```python
from build123d import *

# Parameters (mm, degrees)
F1_DEPTH       = 3.81
F2_R           = 0.254
F3_D           = 1.778
F3_CSINK_D     = 3.175
F3_CSINK_ANGLE = 82


# Not quite as in the source:
# - a feature names something its author has since deleted; it is built from what else it names


with BuildPart() as f1:
    # F0 (on Front) → F1 (new body)
    with BuildSketch(Plane.XZ):
        with BuildLine():
            ThreePointArc((-15.3976073489, 30.0757028162), (-12.6205023663, 18.8138288447), (-15.6854130328, 7.6268524863))
            ThreePointArc((-15.6854130328, 7.6268524863), (-31.3905262472, 3.5144175537), (-39.2854884267, 17.7000537515))
            ThreePointArc((-39.2854884267, 17.7000537515), (-40.2547680717, 20.6965618199), (-43.3147661388, 21.4415285736))
            ThreePointArc((-43.3147661388, 21.4415285736), (-45.5440273695, 15.8957464039), (-45.905020088, 9.9295927212))
            ThreePointArc((-45.905020088, 9.9295927212), (-45.0345404234, 3.597348812), (-45.905020088, -2.7348950971))
            ThreePointArc((-45.905020088, -2.7348950971), (-45.1259294206, -6.5201466433), (-41.5899753571, -8.0796787515))
            Line((-41.5899753571, -8.0796787515), (-40.2320445972, -8.0796787515))
            Line((-40.2320445972, -8.0796787515), (-40.5776619182, -3.1953468446))
            Line((-40.5776619182, -3.1953468446), (-40.0765932374, -1.5246287875))
            Line((-40.0765932374, -1.5246287875), (-40.6392291188, -1.5644411324))
            Line((-40.6392291188, -1.5644411324), (-40.6392291188, 0.5960793933))
            Line((-40.6392291188, 0.5960793933), (-40.0844532998, 0.5960793933))
            Line((-40.0844532998, 0.5960793933), (-40.0844532998, 1.8968694892))
            ThreePointArc((-40.0844532998, 1.8968694892), (-36.1157211919, 2.6708049351), (-32.1480344873, 1.8915278128))
            ThreePointArc((-32.1480344873, 1.8915278128), (-26.4720596319, 0.9912977201), (-20.7960847765, 1.8915278128))
            ThreePointArc((-20.7960847765, 1.8915278128), (-16.7308465178, 3.8739299722), (-13.7448431924, 7.2709675878))
            ThreePointArc((-13.7448431924, 7.2709675878), (-12.3233048625, 12.470180408), (-11.6768007285, 17.821312772))
            ThreePointArc((-11.6768007285, 17.821312772), (-12.1024444853, 23.5936908911), (-13.2695324719, 29.2628555023))
            ThreePointArc((-13.2695324719, 29.2628555023), (-12.6323011565, 32.3319998397), (-9.8052835092, 33.6861349642))
            ThreePointArc((-9.8052835092, 33.6861349642), (-11.5106118889, 35.4421925399), (-12.2696207836, 37.7693772316))
            ThreePointArc((-12.2696207836, 37.7693772316), (-13.3462306374, 38.3418830024), (-13.8277616352, 39.4621416926))
            ThreePointArc((-13.8277616352, 39.4621416926), (-14.9168802382, 39.2283992754), (-15.6854130328, 38.4220667183))
            ThreePointArc((-15.6854130328, 38.4220667183), (-16.3374101507, 34.221439938), (-15.3976073489, 30.0757028162))
        make_face()
    extrude(amount=F1_DEPTH)

    # F2
    f2_edges = [f1.edges().sort_by_distance(p)[0] for p in [
        (-45.90502, -1.905, -2.734895),
        (-13.827762, -1.905, 39.462142),
        (-12.269621, -1.905, 37.769377),
        (-13.346231, 0, 38.341883),
        (-13.346231, -3.81, 38.341883),
        (-11.510612, -3.81, 35.442193),
        (-11.510612, 0, 35.442193),
        (-9.805284, -1.905, 33.686135),
        (-40.232045, -1.905, -8.079679),
    ]]
    fillet(f2_edges, radius=F2_R)

    # F3 (through all)
    with Locations(Plane(origin=(0, 0, 0), x_dir=(1, 0, 0), z_dir=(0, 1, 0))):
        with Locations((-42.347650975, -9.8781445995), (-13.9591796324, -33.550273627)):
            CounterSinkHole(F3_D / 2, F3_CSINK_D / 2, counter_sink_angle=F3_CSINK_ANGLE)


solid = f1.part
```
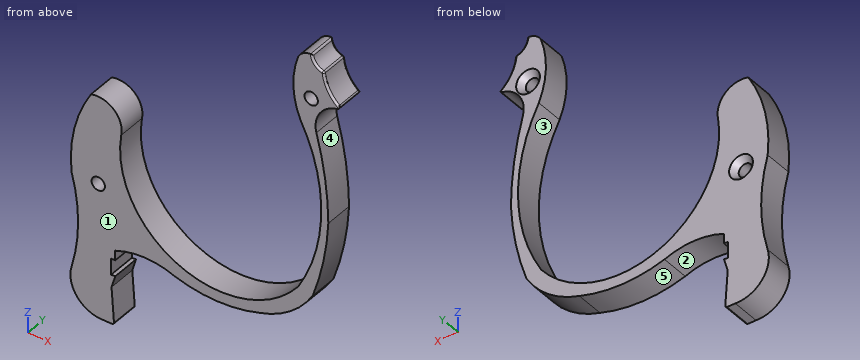
Could you check a few things on this model? Use its own coordinates, in mm. Face numbers are marked on the shaded views. A direction names the side the tool comes from. Coordinates: 2 decimals unless noted, no trailing zeros. Write each loop counter-clockwise with the first axis right and the second up, starting at its lowest first coordinate (ties: lowest second). Pieces come first, ordered by that corner, then holes. Notation, with made-up numbers: M 20.25,53 L 55.25,53 A25 cw 55.25,76 Z; hole C 5,49 d3. An arc over 180 degrees is marked long. Answer as CSV lines item,"result". Start each with the question number.
1) I want a section at B-B, the plane z = 15. Please give me the cut outline in (x, y).
2) I want a section at D-D, the plane y = -1.7. Give the number of separate pieces and of enclosed holes in the cut face, and give its area (3 significant figures).
3) I want a section at C-C, the plane x = -34. Please give me the cut outline in (y, z), and give its area (3 significant figures).
4) I want a section at A-A, the plane z = 5. Please give me the cut outline in (x, y), and give its area (3 significant figures).
5) We'd pull the mould along Z, two halves only. Please class the marked faces 1, 2 and 3: +Z half, -Z half, draft (parallel to the pull), parting line (faces both ways), or undercut.
6) Please list where these lines run through material, in increasing order: line 1 (Z direction, x = -26, y = -0.3); line 2 (Z direction, x = -15, y = -0.75); line 3 (X direction, y = -1.5, z = 15.5). Write a range as from..to.
7) For the marked faces 4 and 5, which set-ups out of +Z, -Z, +X, -X, +Y, -Y let a thin tool reach every point of the face, with its end or its side?
8) For P1, Ø2, axis at x = -13.96, z = 33.55, coming from the +Y side; P2, Ø1.2, axis at x = -41, y = -2, coming from the -Z side; P3, Ø1, axis at y = -2.5, z = 26, coming from the +X side, each with a flat end and sliding along its axis, tell me the tip position at first contact or that it passes through.
Data:
1,outline,"M -45.72,-3.81 L -39.42,-3.81 L -39.42,0 L -45.72,0 Z; M -12.99,-3.81 L -11.92,-3.81 L -11.92,0 L -12.99,0 Z"
2,separate pieces,"1"
2,enclosed holes,"2"
2,area,"287 mm^2"
3,outline,"M -3.81,2.45 L 0,2.45 L 0,5 L -3.81,5 Z"
3,area,"9.69 mm^2"
4,outline,"M -45.08,-3.81 L -34,-3.81 L -34,0 L -45.08,0 Z; M -18.38,-3.81 L -15.46,-3.81 L -15.46,0 L -18.38,0 Z"
4,area,"53.3 mm^2"
5,face 1,"draft"
5,face 2,"-Z half"
5,face 3,"undercut"
6,line 1,"z = 1..2.45"
6,line 2,"z = 5.5..8.91, 29.31..39.18"
6,line 3,"x = -45.63..-39.44, -12.9..-11.86"
7,face 4,"+X, +Y, -Y"
7,face 5,"-Z, +Y, -Y"
8,P1,"stops at y = -0.67"
8,P2,"stops at z = -8.08"
8,P3,"stops at x = -12.41"
